from build123d import *

# Parameters (mm, degrees)
SKETCH1_W           = 63
SKETCH1_H           = 5
BOSS_EXTRUDE1_DEPTH = 30
SKETCH2_W           = 30
SKETCH2_H           = 8
BOSS_EXTRUDE2_DEPTH = 45
SKETCH3_R           = 5
CUT_EXTRUDE1_DEPTH  = 84.030115019
SKETCH5_R           = 1.6
CUT_EXTRUDE3_DEPTH  = 14
FILLET1_R           = 5
BOSS_EXTRUDE3_DEPTH = 30
FILLET2_R           = 2.54
CUT_EXTRUDE5_DEPTH  = 121.258055863
BOSS_EXTRUDE4_REACH = 122.258
SKETCH9_W           = 3.81
SKETCH9_H           = 8.378131559
CHAMFER1_SIZE       = 7.62
SKETCH10_W          = 3.81
SKETCH10_H          = 8.378131559
BOSS_EXTRUDE5_DEPTH = 6
CHAMFER2_SIZE       = 7.62
SKETCH11_W          = 4
SKETCH11_H          = 7
CUT_EXTRUDE6_DEPTH  = 124.616341962
SKETCH13_W          = 10
SKETCH13_H          = 30
BOSS_EXTRUDE6_DEPTH = 2
SKETCH14_R          = 4
BOSS_EXTRUDE7_DEPTH = 10
CHAMFER3_SIZE       = 2
SKETCH15_W          = 30
SKETCH15_H          = 6
CUT_EXTRUDE7_DEPTH  = 1


# Some blends are built 0.0001 mm under size
with BuildPart() as part:
    # Sketch1 → Boss-Extrude1 (new body)
    with BuildSketch(Plane(origin=(0, 0, 0), x_dir=(0, 0, -1), z_dir=(1, 0, 0))):
        with Locations((31.5, 2.5)):
            Rectangle(SKETCH1_W, SKETCH1_H)
    extrude(amount=BOSS_EXTRUDE1_DEPTH)

    # Sketch2 → Boss-Extrude2 (add)
    with BuildSketch(Plane(origin=(0, 5, 0), x_dir=(1, 0, 0), z_dir=(0, 1, 0))):
        with Locations((15, 59)):
            Rectangle(SKETCH2_W, SKETCH2_H)
    extrude(amount=BOSS_EXTRUDE2_DEPTH)

    # Sketch3 → Cut-Extrude1 (cut, through all)
    with BuildSketch(Plane(origin=(0, 5, 0), x_dir=(1, 0, 0), z_dir=(0, 1, 0))):
        with Locations(Location((15, 22, 0), (0, 0, 270))):
            Circle(SKETCH3_R)
    extrude(amount=-CUT_EXTRUDE1_DEPTH, mode=Mode.SUBTRACT)

    # Sketch5 → Cut-Extrude3 (cut)
    with BuildSketch(Plane(origin=(0, 50, 0), x_dir=(1, 0, 0), z_dir=(0, 1, 0))):
        with Locations(Location((5, 59, 0), (0, 0, 270))):
            Circle(SKETCH5_R)
        with Locations(Location((25, 59, 0), (0, 0, 270))):
            Circle(SKETCH5_R)
    extrude(amount=-CUT_EXTRUDE3_DEPTH, mode=Mode.SUBTRACT)

    # Fillet1
    fillet1_edges = [part.edges().sort_by_distance(p)[0] for p in [
        (15, 5, -55),
        (30, 2.5, 0),
        (0, 2.5, 0),
        (15, 0, -63),
    ]]
    fillet(fillet1_edges, radius=FILLET1_R)

    # Sketch6 → Boss-Extrude3 (add)
    with BuildSketch(Plane(origin=(30, 0, 0), x_dir=(0, 0, -1), z_dir=(1, 0, 0))):
        Polygon((63, 41), (63, 37), (105, 37), (105, 15), (63, 15), (63, 11), (109, 11), (109, 41), align=None)
    extrude(amount=-BOSS_EXTRUDE3_DEPTH)

    # Fillet2
    fillet2_edges = [part.edges().sort_by_distance(p)[0] for p in [
        (15, 41, -109),
        (15, 11, -109),
        (15, 11, -63),
        (15, 41, -63),
    ]]
    fillet(fillet2_edges, radius=FILLET2_R)

    # Sketch8 → Cut-Extrude5 (cut, through all)
    with BuildSketch(Plane(origin=(0, 41, 0), x_dir=(1, 0, 0), z_dir=(0, 1, 0))):
        with BuildLine():
            Line((21.793359881, 97.57), (21.793359881, 75.7))
            ThreePointArc((21.793359881, 75.7), (15, 68.906640119), (8.206640119, 75.7))
            Line((8.206640119, 75.7), (8.206640119, 97.57))
            ThreePointArc((8.206640119, 97.57), (15, 104.363359881), (21.793359881, 97.57))
        make_face()
    extrude(amount=-CUT_EXTRUDE5_DEPTH, mode=Mode.SUBTRACT)

    # Boss-Extrude4: up to this face of the body (flat: up to its plane)
    boss_extrude4_end = Plane(part.part.faces().sort_by_distance((15, 50, -59))[0])
    # Sketch9 → Boss-Extrude4 (add, up to the picked face)
    with BuildSketch(Plane(origin=(0, 41, 0), x_dir=(1, 0, 0), z_dir=(0, 1, 0)), mode=Mode.PRIVATE) as boss_extrude4_sk1:
        with Locations((5.715, 67.18906578)):
            Rectangle(SKETCH9_W, SKETCH9_H)
    boss_extrude4_tool1 = split(extrude(boss_extrude4_sk1.sketch, amount=BOSS_EXTRUDE4_REACH, mode=Mode.PRIVATE), bisect_by=boss_extrude4_end, keep=Keep.BOTH, mode=Mode.PRIVATE)
    # Sketch9 → Boss-Extrude4 (add, up to the picked face)
    with BuildSketch(Plane(origin=(0, 41, 0), x_dir=(1, 0, 0), z_dir=(0, 1, 0)), mode=Mode.PRIVATE) as boss_extrude4_sk2:
        with Locations((24.285, 67.18906578)):
            Rectangle(SKETCH9_W, SKETCH9_H)
    boss_extrude4_tool2 = split(extrude(boss_extrude4_sk2.sketch, amount=BOSS_EXTRUDE4_REACH, mode=Mode.PRIVATE), bisect_by=boss_extrude4_end, keep=Keep.BOTH, mode=Mode.PRIVATE)
    add(boss_extrude4_tool1.solids().sort_by(Axis((5.715, 41, -67.189066), (0, 1, 0)))[0])
    add(boss_extrude4_tool2.solids().sort_by(Axis((24.285, 41, -67.189066), (0, 1, 0)))[0])

    # Chamfer1
    chamfer1_edges = [part.edges().sort_by_distance(p)[0] for p in [
        (5.715, 50, -71.378131559),
        (24.285, 50, -71.378131559),
    ]]
    chamfer(chamfer1_edges, length=CHAMFER1_SIZE)

    # Sketch10 → Boss-Extrude5 (add)
    with BuildSketch(Plane.XZ.offset(-11)):
        with Locations((5.715, -67.18906578)):
            Rectangle(SKETCH10_W, SKETCH10_H)
        with Locations((24.285, -67.18906578)):
            Rectangle(SKETCH10_W, SKETCH10_H)
    extrude(amount=BOSS_EXTRUDE5_DEPTH)

    # Chamfer2
    # the kernel refuses this chamfer: 7.62 mm, written as the material it takes off along each edge
    with BuildSketch(Plane(origin=(45.786224368, 5, -71.378131559), x_dir=(0, -0.027495876610586386, 0.9996219169112968), z_dir=(-1, 0, 0))) as chamfer2_piece_1_section:
        Polygon((CHAMFER2_SIZE * 0.999621916911, CHAMFER2_SIZE * 0.0274958766106), (-CHAMFER2_SIZE * 0.0274958766106, CHAMFER2_SIZE * 0.999621916911), (0, 0), align=None)
    chamfer2_piece_1 = extrude(amount=43.002448737, mode=Mode.PRIVATE)
    chamfer2_piece_1 = split(chamfer2_piece_1, bisect_by=Plane(origin=(24.285, 11, -68.732360766), z_dir=(0, -1, 0)), keep=Keep.TOP, mode=Mode.PRIVATE)
    add(chamfer2_piece_1, mode=Mode.SUBTRACT)
    with BuildSketch(Plane(origin=(27.216224368, 5, -71.378131559), x_dir=(0, -0.027495876610586386, 0.9996219169112968), z_dir=(-1, 0, 0))) as chamfer2_piece_2_section:
        Polygon((CHAMFER2_SIZE * 0.999621916911, CHAMFER2_SIZE * 0.0274958766106), (-CHAMFER2_SIZE * 0.0274958766106, CHAMFER2_SIZE * 0.999621916911), (0, 0), align=None)
    chamfer2_piece_2 = extrude(amount=43.002448737, mode=Mode.PRIVATE)
    chamfer2_piece_2 = split(chamfer2_piece_2, bisect_by=Plane(origin=(5.715, 11, -68.732360766), z_dir=(0, -1, 0)), keep=Keep.TOP, mode=Mode.PRIVATE)
    add(chamfer2_piece_2, mode=Mode.SUBTRACT)

    # Sketch11 → Cut-Extrude6 (cut, through all)
    with BuildSketch(Plane(origin=(30, 0, 0), x_dir=(0, 0, -1), z_dir=(1, 0, 0))):
        with Locations((107, 26)):
            Rectangle(SKETCH11_W, SKETCH11_H)
    extrude(amount=-CUT_EXTRUDE6_DEPTH, mode=Mode.SUBTRACT)

    # Sketch13 → Boss-Extrude6 (add)
    with BuildSketch(Plane.ZY):
        with Locations((-94, 26)):
            Rectangle(SKETCH13_W, SKETCH13_H)
    extrude(amount=BOSS_EXTRUDE6_DEPTH)

    # Sketch14 → Boss-Extrude7 (add)
    with BuildSketch(Plane.ZY.offset(2)):
        with Locations((-94, 26)):
            Circle(SKETCH14_R)
    extrude(amount=BOSS_EXTRUDE7_DEPTH)

    # Chamfer3
    chamfer3_edges = [part.edges().sort_by_distance(p)[0] for p in [
        (0, 13, -89),
        (0, 39, -89),
        (0, 13, -99),
        (0, 39, -99),
    ]]
    chamfer(chamfer3_edges, length=CHAMFER3_SIZE - 0.0001)  # a hair under: the kernel refuses the full size

    # Sketch15 → Cut-Extrude7 (cut)
    with BuildSketch(Plane(origin=(0, 41, 0), x_dir=(1, 0, 0), z_dir=(0, 1, 0))):
        with Locations((15, 83)):
            Rectangle(SKETCH15_W, SKETCH15_H)
    extrude(amount=-CUT_EXTRUDE7_DEPTH, mode=Mode.SUBTRACT)


solid = part.part
For this review, take the finished solid that the model builds, in its own axes (mm). A direction names the side the tool comes from. Give positions to 0.01 mm unless a question says otherwise; leave off trailing zeros. Loops run counter-clockwise (first coordinate to the right, second up) from the corner with the lowest first, then second, coordinate; pieces in that order, holes last. Notation, with made-up numbers: M -27.5,17.25 L 11.5,17.25 A35 ccw 11.5,49.25 Z; hole C 43,43.25 d5. An arc over 180 degrees is marked long. Answer as a JSON object with one key per item and string values. Group by question number.
Q1. Mouldability with a two-part tool opening along X and no side actions: class faces 4 (the flat face through (-2, 30, -96)), 5 (the flat face through (5, 36, -59)), 6 (the cylindrical face through (15, 7, -54)) as +X half, -X half, draft (parallel to the pull), parting line (faces both ways), or undercut.
Q2. For probe 1 along X at (y, z) = (41, -59); probe 2 along Z at (x, y) = (3.5, 34); probe 3 along Y at (x, z) = (21, -67.5), list the stretches that pass through material, from the lowest coordinate up. Write a range as [from, to].
Q3. Add section C-C on z = -94. Give the boundary of the cut face in (x, y).
Q4. Add section D-D on y = 18. Give the boundary of the cut face in (x, z), and give its area (3 significant figures).
Q5. Add section A-A on z = -22. Give the boundary of the cut face in (x, y), and give its area (3 significant figures).
Q6. Add section B-B on y = 26. Give the boundary of the cut face in (x, z).
Q7. Insertion check: P1, Ø1, axis at x = 2, y = 43.5, coming from the -Z side; P2, Ø6.5, axis at y = 46.5, z = -68, coming from the -X side; P3, Ø1.6, axis at x = 5.5, z = -59.5, coming from the +Y side. Each pin has a flat end and moves straight along its axis. Give the tip position at first contact, or say it passes through.
Q8. Tool access review of faces 1 (the flat face through (7, 37, -84)), 2 (the cylindrical face through (-6.93, 28.7, -96.95)), 3 (the flat face through (26, 40, -83)): name each direction out of +Z, -Z, +X, -X, +Y, -Y from which nothing blocks a thin tool from reaching the whole face with its end or side.
Checked values:
{
 "1": {"face 4": "-X half", "face 5": "undercut", "face 6": "draft"},
 "2": {"probe 1": "[0, 3.4], [6.6, 23.4], [26.6, 30]", "probe 2": "[-109, -105], [-63, -55]", "probe 3": "[11, 15], [37, 41]"},
 "3": {"outline": "M -12,22 L -2,22 L -2,11 L 8.21,11 L 8.21,15 L 0,15 L 0,37 L 8.21,37 L 8.21,41 L -2,41 L -2,30 L -12,30 Z; M 21.79,11 L 30,11 L 30,15 L 21.79,15 Z; M 21.79,37 L 30,37 L 30,41 L 21.79,41 Z"},
 "4": {"outline": "M -2,-99 L 0,-99 L 0,-89 L -2,-89 Z; M 0,-109 L 30,-109 L 30,-105 L 0,-105 Z; M 0,-63 L 30,-63 L 30,-55 L 0,-55 Z", "area": "380 mm²"},
 "5": {"outline": "M 0,0 L 10,0 L 10,5 L 0,5 Z; M 20,0 L 30,0 L 30,5 L 20,5 Z", "area": "100 mm²"},
 "6": {"outline": "M -12,-98 L -2,-98 L -2,-99 L 0,-99 L 0,-89 L -2,-89 L -2,-90 L -12,-90 Z; M 0,-63 L 30,-63 L 30,-55 L 0,-55 Z"},
 "7": {"P1": "z = -63.06", "P2": "x = 3.81", "P3": "y = 36"},
 "8": {"face 1": "+X", "face 2": "-X", "face 3": "+X, -X, +Y"}
}
